Verification items for the finished model (mm, model axes). Face numbers are marked on the shaded views. Round coordinates to 2 decimals unless told otherwise and drop trailing zeros. Order: outer loops, then holes, each group sorted by start corner. A loop starts at its lowest first (then second) coordinate and runs counter-clockwise, first axis right, second up. Notation, with made-up numbers: (-12.75, 17.25) -> (-7.75, 17.25) arc R17 cw to (-7.75, 23.25) -> close; hole circle Ø1 at (15.25, -15). An arc over 180 degrees is marked (long way). Return JSON: item names as keys, results as strings. Group by question number.
Item 1: Sectioned sample at C-C on y = 30. Record the cut outline in (x, z), plus the area to 3 significant figures.
Item 2: Draft check along Y on the marked faces 1, 2 and 3. Enter one of: pulls with the +Y half, pulls with the -Y half, needs draft (parallel to the pull), parting line crosses it, or undercut.
Item 3: Sectioned sample at D-D on z = 3.5. Give the number of separate pieces and of enclosed holes in the cut face, plus the area to 3 significant figures.
Item 4: Scan lines: probe 1 along X at (y, z) = (30, 0.5); probe 2 along X at (y, z) = (28, 3); probe 3 along Y at (x, z) = (-49.5, 3.5). Record each from-to range of solid material in increasing order. Write a range as from..to.
Item 5: Sectioned sample at B-B on y = 49. Record the cut outline in (x, z).
Item 6: Depth check by flat-ended pin: pin 1 Ø2 at (y, z) = (50, 1) entering from +X; pin 2 Ø1 at (x, z) = (-51.5, 5) entering from +Y. Enter the tip coordinate at first touch or a pass-through.
Item 7: Sectioned sample at A-A on x = -61. Record the cut outline in (y, z).
```python
from build123d import *

# Parameters (mm, degrees)
F0_R     = 6.35
F1_DEPTH = 6.35


with BuildPart() as f1:
    # F0 (on Top) → F1 (new body)
    with BuildSketch(Plane.XY):
        with BuildLine():
            ThreePointArc((-53.1782564477, 41.6842693984), (-48.3327406635, 45.1317048361), (-46.4763714082, 50.7812824752))
            ThreePointArc((-46.4763714082, 50.7812824752), (-47.3162680415, 54.6921141654), (-49.6878369219, 57.9132462503))
            ThreePointArc((-49.6878369219, 57.9132462503), (-58.4100557825, 59.9966969849), (-64.9972519962, 53.911738903))
            Line((-64.9972519962, 53.911738903), (-65.2636588151, 53.0029163317))
            ThreePointArc((-65.2636588151, 53.0029163317), (-62.5124141472, 43.8291642763), (-53.1782564477, 41.6842693984))
        make_face()
        with Locations((-56.0013714082, 50.7812824752)):
            Circle(F0_R, mode=Mode.SUBTRACT)
        with BuildLine():
            Line((-65.2636588151, 53.0029163317), (-64.9972519962, 53.911738903))
            ThreePointArc((-64.9972519962, 53.911738903), (-65.1417578469, 53.4606407474), (-65.2636588151, 53.0029163317))
        make_face()
        with BuildLine():
            ThreePointArc((-21.8725080792, 30.7135868106), (-22.7936822086, 34.8001263475), (-25.3790288954, 38.096237643))
            ThreePointArc((-25.3790288954, 38.096237643), (-35.0554610731, 39.5081877051), (-40.8763247582, 31.6504215705))
            ThreePointArc((-40.8763247582, 31.6504215705), (-38.1559117236, 24.0016865446), (-30.5261420942, 21.2285277006))
            ThreePointArc((-30.5261420942, 21.2285277006), (-24.3609824448, 24.29385691), (-21.8725080792, 30.7135868106))
        make_face()
        with Locations((-31.3975080792, 30.7135868106)):
            Circle(F0_R, mode=Mode.SUBTRACT)
        with BuildLine():
            ThreePointArc((-55.3962625933, 20.3100166458), (-55.9742861224, 23.5776208185), (-57.638202127, 26.4486366246))
            ThreePointArc((-57.638202127, 26.4486366246), (-66.8844329452, 29.6305095066), (-74.061649032, 22.989374918))
            ThreePointArc((-74.061649032, 22.989374918), (-71.5818043374, 13.5009925839), (-62.0410610516, 11.2309162454))
            ThreePointArc((-62.0410610516, 11.2309162454), (-57.2349258623, 14.6845519842), (-55.3962625933, 20.3100166458))
        make_face()
        with Locations((-64.9212625933, 20.3100166458)):
            Circle(F0_R, mode=Mode.SUBTRACT)
        with BuildLine():
            ThreePointArc((-57.638202127, 26.4486366246), (-59.4965211645, 35.2632237636), (-53.1782564477, 41.6842693984))
            ThreePointArc((-53.1782564477, 41.6842693984), (-62.5124141472, 43.8291642763), (-65.2636588151, 53.0029163317))
            Line((-65.2636588151, 53.0029163317), (-74.061649032, 22.989374918))
            ThreePointArc((-74.061649032, 22.989374918), (-66.8844329452, 29.6305095066), (-57.638202127, 26.4486366246))
        make_face()
        with BuildLine():
            ThreePointArc((-49.6878369219, 57.9132462503), (-47.3162680415, 54.6921141654), (-46.4763714082, 50.7812824752))
            ThreePointArc((-46.4763714082, 50.7812824752), (-48.3327406635, 45.1317048361), (-53.1782564477, 41.6842693984))
            ThreePointArc((-53.1782564477, 41.6842693984), (-44.7055638187, 40.2558870979), (-40.8301414364, 32.5872563373))
            ThreePointArc((-40.8301414364, 32.5872563373), (-40.841694273, 32.1182701223), (-40.8763247582, 31.6504215705))
            ThreePointArc((-40.8763247582, 31.6504215705), (-35.0554610731, 39.5081877051), (-25.3790288954, 38.096237643))
            Line((-25.3790288954, 38.096237643), (-49.6878369219, 57.9132462503))
        make_face()
        with BuildLine():
            ThreePointArc((-40.8763247582, 31.6504215705), (-47.5320265353, 23.4902432421), (-57.638202127, 26.4486366246))
            ThreePointArc((-57.638202127, 26.4486366246), (-55.9742861224, 23.5776208185), (-55.3962625933, 20.3100166458))
            ThreePointArc((-55.3962625933, 20.3100166458), (-57.2349258623, 14.6845519842), (-62.0410610516, 11.2309162454))
            Line((-62.0410610516, 11.2309162454), (-30.5261420942, 21.2285277006))
            ThreePointArc((-30.5261420942, 21.2285277006), (-38.1559117236, 24.0016865446), (-40.8763247582, 31.6504215705))
        make_face()
        with BuildLine():
            ThreePointArc((-40.8301414364, 32.5872563373), (-44.7055638187, 40.2558870979), (-53.1782564477, 41.6842693984))
            ThreePointArc((-53.1782564477, 41.6842693984), (-59.4965211645, 35.2632237636), (-57.638202127, 26.4486366246))
            ThreePointArc((-57.638202127, 26.4486366246), (-47.5320265353, 23.4902432421), (-40.8763247582, 31.6504215705))
            ThreePointArc((-40.8763247582, 31.6504215705), (-40.841694273, 32.1182701223), (-40.8301414364, 32.5872563373))
        make_face()
        with Locations((-50.3551414364, 32.5872563373)):
            Circle(F0_R, mode=Mode.SUBTRACT)
    extrude(amount=F1_DEPTH)


solid = f1.part
```
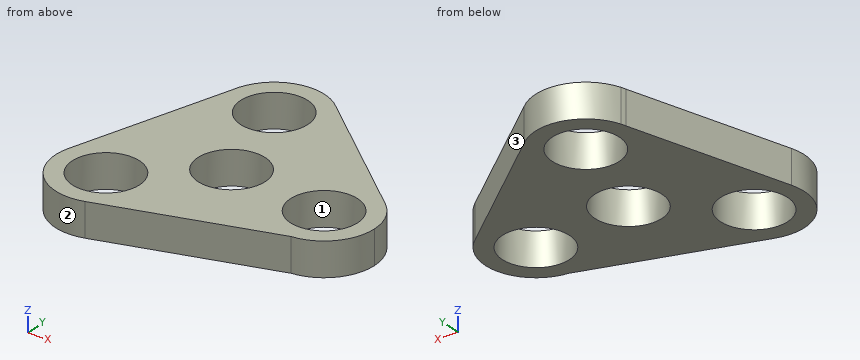
Recorded:
{
 "1": {"outline": "(-72.01, 0) -> (-56.15, 0) -> (-56.15, 6.35) -> (-72.01, 6.35) -> close; (-44.56, 0) -> (-37.71, 0) -> (-37.71, 6.35) -> (-44.56, 6.35) -> close; (-25.09, 0) -> (-21.9, 0) -> (-21.9, 6.35) -> (-25.09, 6.35) -> close", "area": "164 mm²"},
 "2": {"face 1": "undercut", "face 2": "parting line crosses it", "face 3": "pulls with the +Y half"},
 "3": {"separate pieces": "1", "enclosed holes": "4", "area": "1,180 mm²"},
 "4": {"probe 1": "-72.01..-56.15, -44.56..-37.71, -25.09..-21.9", "probe 2": "-72.59..-54.75, -45.96..-37.14, -25.66..-22.27", "probe 3": "15.21..26.3, 38.88..57.76"},
 "5": {"outline": "(-66.44, 0) -> (-62.1, 0) -> (-62.1, 6.35) -> (-66.44, 6.35) -> close; (-49.91, 0) -> (-38.75, 0) -> (-38.75, 6.35) -> (-49.91, 6.35) -> close"},
 "6": {"pin 1": "x = -38.75", "pin 2": "y = 59.43"},
 "7": {"outline": "(11.56, 0) -> (15.32, 0) -> (15.32, 6.35) -> (11.56, 6.35) -> close; (25.3, 0) -> (46.87, 0) -> (46.87, 6.35) -> (25.3, 6.35) -> close; (54.7, 0) -> (58.89, 0) -> (58.89, 6.35) -> (54.7, 6.35) -> close"}
}
